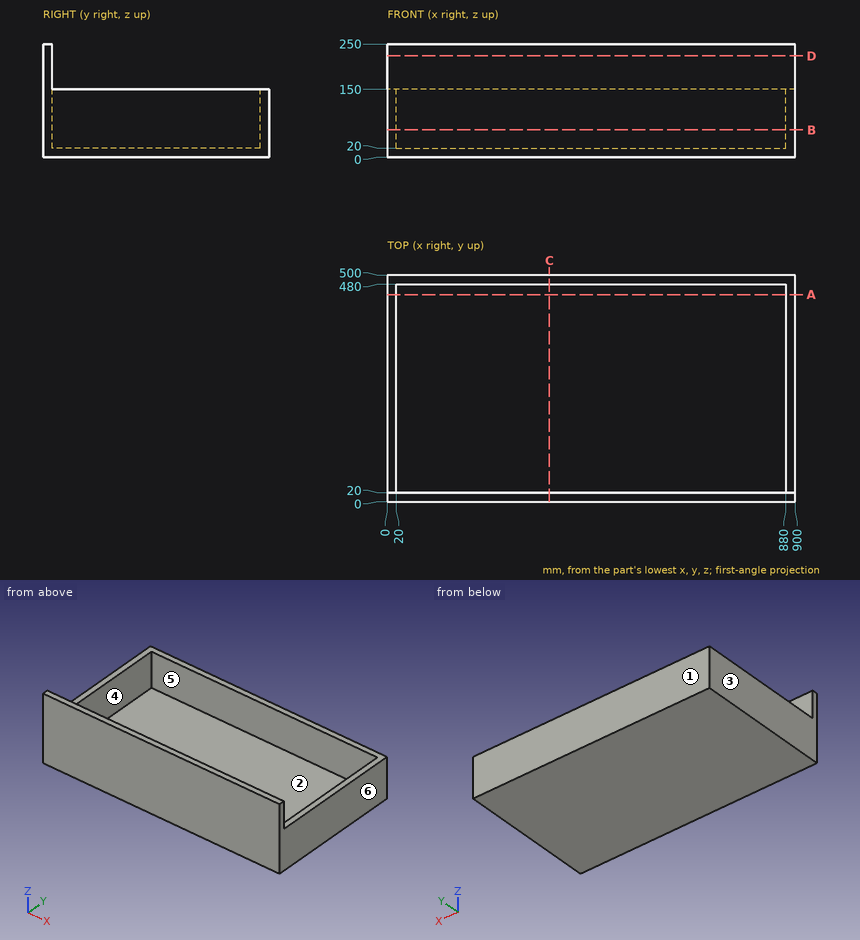
Answer from the drawing. Dimensions are ordinates in mm from the lowest x, y and z of the part. A direction names the side the tool comes from. Coordinates: 2 decimals unless noted, no trailing zeros. Order: outer loops, then holes, each group sorted by start corner. A loop starts at its lowest first (then second) coordinate and runs counter-clockwise, first axis right, second up. Notation, with made-up numbers: M 13,-3.75 L 40,-3.75 A16 ccw 40,26.25 Z; hole C 19,-11 d7. An arc over 180 degrees is marked long. Put each result on its own line as item: value. Start each with the question number.
Item 1: The mould has two halves that part along X. Classify the marked faces 3, 4, 5 and 6: +X half, -X half, draft (parallel to the pull), parting line (faces both ways), or undercut.
Item 2: Given pin 1 Ø10 at (x, z) = (271.5, 211) entering from +Y; pin 2 Ø12 at (x, z) = (338.5, 40.5) entering from -Y; pin 3 Ø1.5 at (x, y) = (798.5, 198) entering from +Z, each flat-ended and moving along its own axis, determine where each tip first touches the part or whether it passes through.
Item 3: Section A-A, the plane y = 457 is taken. Determine the outline of the cut face in (x, z).
Item 4: For the marked faces 1 and 2, determine the directions among +Z, -Z, +X, -X, +Y, -Y from which every point of the face is accessible in a straight line to the end or side of a thin tool.
Item 5: Section D-D, the plane z = 224 is taken. Determine the outline of the cut face in (x, y).
Item 6: Section C-C, the plane x = 357.5 is taken. Determine the outline of the cut face in (y, z).
Item 7: Section B-B, the plane z = 60.5 is taken. Determine the outline of the cut face in (x, y), plus the area to 3 significant figures.
Item 8: Consider probe 1 along X at (y, z) = (167, 94); probe 2 along Y at (x, z) = (661, 68.5); probe 3 along Z at (x, y) = (203.5, 314.5). Determine where each line is inside the solid, lowest interval first. Write a range as [from, to].
Computed:
1. face 3: -X half
1. face 4: undercut
1. face 5: undercut
1. face 6: +X half
2. pin 1: stops at y = 20
2. pin 2: stops at y = 0
2. pin 3: stops at z = 20
3. outline: M 0,0 L 900,0 L 900,150 L 880,150 L 880,20 L 20,20 L 20,150 L 0,150 Z
4. face 1: +Z, -Z, +X, -X, +Y
4. face 2: +Z
5. outline: M 0,0 L 900,0 L 900,20 L 0,20 Z
6. outline: M 0,0 L 500,0 L 500,150 L 480,150 L 480,20 L 20,20 L 20,250 L 0,250 Z
7. outline: M 0,0 L 900,0 L 900,500 L 0,500 Z; hole M 20,20 L 880,20 L 880,480 L 20,480 Z
7. area: 54,400 mm2
8. probe 1: x = [0, 20], [880, 900]
8. probe 2: y = [0, 20], [480, 500]
8. probe 3: z = [0, 20]
